Can you work these out from the model? Positions are in its coordinate system, mm. Give positions to 0.01 mm unless a question says otherwise; leave off trailing zeros. Order: outer loops, then holes, each group sorted by start corner. A loop starts at its lowest first (then second) coordinate and runs counter-clockwise, first axis right, second up. Notation, with made-up numbers: M 27,49 L 73,49 A28 cw 73,81 Z; hole C 15,60.5 d9. An arc over 180 degrees is marked long. Answer as a JSON object with one key per item and string values.
```python
from build123d import *

# Parameters (mm, degrees)
FILLET1_R = 0.142875


with BuildPart() as part:
    # Sketch2 → Revolve1 (revolve)
    with BuildSketch(Plane.XY):
        Polygon((-7.34375, -4.88975), (-7.34375, 6.7625), (-4.7625, 6.7625), (-4.7625, -0.79375), (0.2375, -0.79375), (0.2375, -4.88975), align=None)
    revolve(axis=Axis((0.2375, -0.79375, 0), (0, -1, 0)))

    # Fillet1
    fillet1_edges = [part.edges().sort_by_distance(p)[0] for p in [
        (5.2375, 6.7625, 0),
        (7.81875, 6.7625, 0),
    ]]
    fillet(fillet1_edges, radius=FILLET1_R)


solid = part.part
```
1) Thinking about a two-plate mould opening in X: for faces 1 (the face through (-4.532, 2.861, -1.502)), 2 (the face through (0, -4.89, 0)), 3 (the face through (7.81, 0.95, -0.33)), 4 (the face through (0, -0.794, 0)), which applies, pulls with the +X half, pulls with the -X half, needs draft (parallel to the pull), parting line crosses it, or undercut?
Results found:
{"face 1": "undercut", "face 2": "needs draft", "face 3": "parting line crosses it", "face 4": "undercut"}
2) I'm going to push flat-ended pins straight in: pin 1 Ø2 at (x, y) = (-4, -1.5) entering from +Z; pin 2 Ø3 at (x, y) = (2, 3) entering from -Z; pin 3 Ø1.5 at (y, z) = (0.5, 6) entering from +X; pin 4 Ø5 at (x, z) = (2, -2) entering from +Y. Where does each tip first touch, or does it pass through?
Results found:
{"pin 1": "stops at z = 6.86", "pin 2": "stops at z = -7.58", "pin 3": "stops at x = 5.71", "pin 4": "stops at y = 6.76"}
3) I want a section at C-C on y = -2. Write out the boundary of the cut face in (x, z), and give its area (3 significant figures).
Results found:
{"outline": "C 0.24,0 d15.16", "area": "181 mm²"}
4) I want a section at A-A on z = 0. Write out the boundary of the cut face in (x, y), and give its area (3 significant figures).
Results found:
{"outline": "M -7.34,-4.89 L 7.82,-4.89 L 7.82,6.62 A0.14 ccw 7.68,6.76 L 5.38,6.76 A0.14 ccw 5.24,6.62 L 5.24,-0.79 L -4.76,-0.79 L -4.76,6.62 A0.14 ccw -4.91,6.76 L -7.2,6.76 A0.14 ccw -7.34,6.62 Z", "area": "101 mm²"}
5) I want a section at B-B on y = 1. Write out the boundary of the cut face in (x, z), and give its area (3 significant figures).
Results found:
{"outline": "C 0.24,0 d15.16; hole C 0.24,0 d10", "area": "102 mm²"}
6) I need wall thicknesses on L1, parallel to X at y = 2.25, z = 0; L2, parallel to Y at x = 4.25, z = 2.5; L3, parallel to X at y = 6, z = -1.75. Which ranges of each line are inside material? Lowest first, please.
Results found:
{"L1": "x = -7.34 to -4.76, 5.24 to 7.82", "L2": "y = -4.89 to -0.79", "L3": "x = -7.14 to -4.45, 4.92 to 7.61"}
